Source: CAD feature listing. Evaluate the final solid. Frame: model axes, mm. A direction names the side the tool comes from. Give positions to 0.01 mm unless a question says otherwise; leave off trailing zeros. Order: outer loops, then holes, each group sorted by start corner. A loop starts at its lowest first (then second) coordinate and runs counter-clockwise, first axis right, second up. Notation, with made-up numbers: M 7.25,-7 L 19.25,-7 A24 cw 19.25,7 Z; hole C 12,39.25 d7. An arc over 180 degrees is marked long. Return JSON: item names as keys, results as strings.
from build123d import *

# Parameters (mm, degrees)
SKETCH1_W           = 150
SKETCH1_H           = 100
BOSS_EXTRUDE1_DEPTH = 15
SKETCH2_R           = 5
CUT_EXTRUDE2_DEPTH  = 15
SKETCH4_R           = 10
BOSS_EXTRUDE3_DEPTH = 7.5
BOSS_EXTRUDE4_DEPTH = 7.5
BOSS_EXTRUDE5_DEPTH = 7.5


with BuildPart() as part:
    # Sketch1 → Boss-Extrude1 (new body)
    with BuildSketch(Plane(origin=(0, 0, 0), x_dir=(1, 0, 0), z_dir=(0, 1, 0))):
        Rectangle(SKETCH1_W, SKETCH1_H)
    extrude(amount=BOSS_EXTRUDE1_DEPTH)

    # Sketch2 → Cut-Extrude2 (cut)
    with BuildSketch(Plane(origin=(0, 15, 0), x_dir=(1, 0, 0), z_dir=(0, 1, 0))):
        with Locations((45, -30)):
            Circle(SKETCH2_R)
        with Locations((45, 30)):
            Circle(SKETCH2_R)
        with Locations((-45, 30)):
            Circle(SKETCH2_R)
        with Locations((-45, -30)):
            Circle(SKETCH2_R)
    extrude(amount=-CUT_EXTRUDE2_DEPTH, mode=Mode.SUBTRACT)

    # Sketch4 → Boss-Extrude3 (add, symmetric)
    with BuildSketch(Plane.XY):
        with BuildLine():
            Line((75, 15), (-75, 15))
            Line((-75, 15), (-144.282032303, 55))
            ThreePointArc((-144.282032303, 55), (-154.13052805, 87.855309915), (-121.911493446, 99.61958071))
            Line((-121.911493446, 99.61958071), (75, 15))
        make_face()
        with Locations((-131.782032303, 76.650635095)):
            Circle(SKETCH4_R, mode=Mode.SUBTRACT)
    extrude(amount=BOSS_EXTRUDE3_DEPTH, both=True)

    # Sketch5 → Boss-Extrude4 (add, symmetric)
    with BuildSketch(Plane(origin=(0, 0, 0), x_dir=(0, 0, -1), z_dir=(1, 0, 0))):
        Polygon((-7.5, 15), (-7.5, 35), (-50, 15), align=None)
    extrude(amount=BOSS_EXTRUDE4_DEPTH, both=True)

    # Sketch6 → Boss-Extrude5 (add, symmetric)
    with BuildSketch(Plane(origin=(0, 0, 0), x_dir=(0, 0, -1), z_dir=(1, 0, 0))):
        Polygon((7.5, 15), (7.5, 35), (50, 15), align=None)
    extrude(amount=BOSS_EXTRUDE5_DEPTH, both=True)


solid = part.part
1. Ray query, probe 1 along Z at (x, y) = (45, 7.5); probe 2 along X at (y, z) = (9, -30); probe 3 along Y at (x, z) = (44, -11). Return the intervals inside material, ascending.
Evaluation:
{"probe 1": "z = -50 to -35, -25 to 25, 35 to 50", "probe 2": "x = -75 to -50, -40 to 40, 50 to 75", "probe 3": "y = 0 to 15"}
2. Draft query along Z for faces 1 (the face through (0.11, 25.14, 28.45)), 2 (the face through (-50, 8, 30)), 3 (the face through (-75, 7, 1)). Return one class per face: pulls with the +Z half, pulls with the -Z half, needs draft (parallel to the pull), parting line crosses it, or undercut.
Evaluation:
{"face 1": "pulls with the +Z half", "face 2": "undercut", "face 3": "needs draft"}
3. Section query A-A (x = 45). Return loops of the section in (y, z), then the cut area to 3 significant figures.
Evaluation:
{"outline": "M 0,-50 L 15,-50 L 15,-35 L 0,-35 Z; M 0,-25 L 15,-25 L 15,-7.5 L 27.89,-7.5 L 27.89,7.5 L 15,7.5 L 15,25 L 0,25 Z; M 0,35 L 15,35 L 15,50 L 0,50 Z", "area": "1,390 mm^2"}
4. Set-up query: faces 4 (the face through (-7.5, 21, 20)), 5 (the face through (-7.5, 21, -20)), 6 (the face through (7.5, 21, 20)), 7 (the face through (41, 15, -24)). Return all of +Z, -Z, +X, -X, +Y, -Y with unobstructed straight access to the full face (end or side cutting, diameter ignored); none if empty.
Evaluation:
{"face 4": "+Z, -X, +Y", "face 5": "-Z, -X, +Y", "face 6": "+Z, +X, +Y", "face 7": "-Z, +X, +Y"}
5. Section query D-D (x = -60). Return loops of the section in (y, z).
Evaluation:
{"outline": "M 0,-50 L 15,-50 L 15,-7.5 L 73.01,-7.5 L 73.01,7.5 L 15,7.5 L 15,50 L 0,50 Z"}
6. Section query B-B (y = 79.5). Return loops of the section in (x, z).
Evaluation:
{"outline": "M -156.62,-7.5 L -141.37,-7.5 L -141.37,7.5 L -156.62,7.5 Z; M -122.2,-7.5 L -75.09,-7.5 L -75.09,7.5 L -122.2,7.5 Z"}
7. Section query C-C (z = 30). Return loops of the section in (x, y).
Evaluation:
{"outline": "M -75,0 L -50,0 L -50,15 L -75,15 Z; M -40,0 L 40,0 L 40,15 L 7.5,15 L 7.5,24.41 L -7.5,24.41 L -7.5,15 L -40,15 Z; M 50,0 L 75,0 L 75,15 L 50,15 Z"}
8. First-contact query: pin 1 (22 mm diameter, centred on y = 29.5, z = 37, fed in from -X); pin 2 (13 mm diameter, centred on x = 52, z = 38.5, fed in from +Y); pin 3 (8 mm diameter, centred on y = 42, z = -3, fed in from +X). Flat tips, straight axial feed; report the tip coordinate or a pass-through.
Evaluation:
{"pin 1": "stops at x = -7.5", "pin 2": "stops at y = 15", "pin 3": "stops at x = 21.48"}
